Input: part model. Units: mm. Frame: model coordinates. A direction names the side the tool comes from. Round coordinates to 2 decimals unless told otherwise and drop trailing zeros. Order: outer loops, then holes, each group sorted by start corner. A loop starts at its lowest first (then second) coordinate and runs counter-clockwise, first axis right, second up. Notation, with made-up numbers: (57, 12) -> (82, 12) arc R21 ccw to (82, 32) -> close; hole circle Ø9 at (-10.5, 88.25). An arc over 180 degrees is marked (long way). Use a Markdown table: item, result.
from build123d import *

# Parameters (mm, degrees)
F0_W      = 72
F0_H      = 132
F1_DEPTH  = 13
F2_W      = 66
F2_H      = 126
F3_DEPTH  = 8.5
F4_W      = 72
F4_H      = 132
F4_W_2    = 66
F4_H_2    = 126
F4_W_3    = 63
F4_H_3    = 123
F5_DEPTH  = 1.2
F6_R      = 7.5
F7_DEPTH  = 25
F8_DEPTH  = 25
F9_R      = 5
F10_DEPTH = 25
F11_W     = 14
F11_H     = 6.5
F12_DEPTH = 25
F13_W     = 35
F13_H     = 3
F14_DEPTH = 25
F15_W     = 95.4631343484
F15_H     = 107.6438874006
F16_DEPTH = 14.201


with BuildPart() as f1:
    # F0 (on Front) → F1 (new body)
    with BuildSketch(Plane.XZ):
        Rectangle(F0_W, F0_H)
    extrude(amount=F1_DEPTH)

    # F2 (on face) → F3 (cut)
    with BuildSketch(Plane.XZ.offset(13)):
        Rectangle(F2_W, F2_H)
    extrude(amount=-F3_DEPTH, mode=Mode.SUBTRACT)

    # F4 (on face) → F5 (join)
    with BuildSketch(Plane.XZ.offset(13)):
        Rectangle(F4_W, F4_H)
        Rectangle(F4_W_2, F4_H_2, mode=Mode.SUBTRACT)
        Rectangle(F4_W_2, F4_H_2)
        Rectangle(F4_W_3, F4_H_3, mode=Mode.SUBTRACT)
    extrude(amount=F5_DEPTH)

    # F6 (on face) → F7 (cut)
    with BuildSketch(Plane.XZ.offset(4.5)):
        with Locations((0, 50)):
            Circle(F6_R)
    extrude(amount=-F7_DEPTH, mode=Mode.SUBTRACT)

    # F6 (on face) → F8 (cut)
    with BuildSketch(Plane.XZ.offset(4.5)):
        with Locations((0, 50)):
            Circle(F6_R)
    extrude(amount=-F8_DEPTH, mode=Mode.SUBTRACT)

    # F9 (on face) → F10 (cut)
    with BuildSketch(Plane.XZ.offset(4.5)):
        with Locations((0, 39.799913764)):
            Circle(F9_R)
    extrude(amount=-F10_DEPTH, mode=Mode.SUBTRACT)

    # F11 (on face) → F12 (cut)
    with BuildSketch(Plane.XY.offset(66)):
        with Locations((0, -7.45)):
            Rectangle(F11_W, F11_H)
    extrude(amount=-F12_DEPTH, mode=Mode.SUBTRACT)

    # F13 (on face) → F14 (cut)
    with BuildSketch(Plane.XZ.offset(4.5)):
        with Locations((0, -54)):
            Rectangle(F13_W, F13_H)
    extrude(amount=-F14_DEPTH, mode=Mode.SUBTRACT)

    # F15 (on Front) → F16 (cut, through all)
    with BuildSketch(Plane.XZ):
        with Locations((-3.6825537682, -16.5714919567)):
            Rectangle(F15_W, F15_H)
    extrude(amount=F16_DEPTH, mode=Mode.SUBTRACT)


solid = f1.part
1) Pull-direction query (Y, two-part tool) for faces 5 (the flat face through (33, -9, 50)), 6 (the flat face through (-1, 0, 58)), 7 (the flat face through (23, -4, 37.25)); classes: +Y half, -Y half, draft (parallel to the pull), parting line (faces both ways), or undercut.
Results found:
| item | result |
|---|---|
| face 5 | undercut |
| face 6 | +Y half |
| face 7 | draft |
2) Cut plane C-C on x = 0. Return loops of the section in (y, z).
Results found:
| item | result |
|---|---|
| outline | (-14.2, 61.5) -> (-13, 61.5) -> (-13, 63) -> (-10.7, 63) -> (-10.7, 66) -> (-14.2, 66) -> close; (-4.2, 57.5) -> (0, 57.5) -> (0, 66) -> (-4.2, 66) -> close |
3) Cut plane A-A on y = -6.5. Return loops of the section in (x, z), and give its area (3 significant figures).
Results found:
| item | result |
|---|---|
| outline | (-36, 37.25) -> (-33, 37.25) -> (-33, 63) -> (-7, 63) -> (-7, 66) -> (-36, 66) -> close; (7, 63) -> (33, 63) -> (33, 37.25) -> (36, 37.25) -> (36, 66) -> (7, 66) -> close |
| area | 328 mm² |
4) Set-up query: faces 1 (the flat face through (31.5, -14, 49)), 2 (the flat face through (-33, -9, 50)), 3 (the flat face through (6, -4.2, 43)), 4 (the cylindrical face through (4.964, -2.282, 40.401)). Return all of +Z, -Z, +X, -X, +Y, -Y with unobstructed straight access to the full face (end or side cutting, diameter ignored); none if empty.
Results found:
| item | result |
|---|---|
| face 1 | -Z, -Y |
| face 2 | -Z |
| face 3 | +Z, -Y |
| face 4 | +Y, -Y |
5) Pin query (flat end, axial travel): pin 1 Ø3 at (x, y) = (-15, -12.5) entering from -Z; pin 2 Ø4 at (x, y) = (16, -9.5) entering from -Z; pin 3 Ø7.5 at (x, z) = (-12, 46.5) entering from -Y. Return the tip coordinate at first contact, or that it passes through.
Results found:
| item | result |
|---|---|
| pin 1 | stops at z = 61.5 |
| pin 2 | stops at z = 63 |
| pin 3 | stops at y = -4.5 |
6) Line query: L1, parallel to X at y = -8.75, z = 52; L2, parallel to X at y = -1.55, z = 50; L3, parallel to Y at x = -29, z = 49. Output: solid intervals per line, ascending. Write a range as [from, to].
Results found:
| item | result |
|---|---|
| L1 | x = [-36, -33], [33, 36] |
| L2 | x = [-36, -7.5], [7.5, 36] |
| L3 | y = [-4.5, 0] |
7) Cut plane B-B on z = 50. Return loops of the section in (x, y).
Results found:
| item | result |
|---|---|
| outline | (-36, -14.2) -> (-31.5, -14.2) -> (-31.5, -13) -> (-33, -13) -> (-33, -4.5) -> (-7.5, -4.5) -> (-7.5, 0) -> (-36, 0) -> close; (7.5, -4.5) -> (33, -4.5) -> (33, -13) -> (31.5, -13) -> (31.5, -14.2) -> (36, -14.2) -> (36, 0) -> (7.5, 0) -> close |
8) Cut plane D-D on z = 60. Return loops of the section in (x, y), and give its area (3 significant figures).
Results found:
| item | result |
|---|---|
| outline | (-36, -14.2) -> (-31.5, -14.2) -> (-31.5, -13) -> (-33, -13) -> (-33, -4.5) -> (-7, -4.5) -> (-7, -4.2) -> (7, -4.2) -> (7, -4.5) -> (33, -4.5) -> (33, -13) -> (31.5, -13) -> (31.5, -14.2) -> (36, -14.2) -> (36, 0) -> (-36, 0) -> close |
| area | 382 mm² |
